Part print with two shaded views. Sizes in mm from the minimum x, y, z corner. A direction names the side the tool comes from. Give positions to 0.01 mm unless a question says otherwise; leave off trailing zeros. Order: outer loops, then holes, each group sorted by start corner. A loop starts at its lowest first (then second) coordinate and runs counter-clockwise, first axis right, second up. Notation, with made-up numbers: M -36,11.5 L -10,11.5 A23 cw -10,48.5 Z; hole C 21.25,65 d1. An arc over 180 degrees is marked long. Answer as CSV lines item,"result".
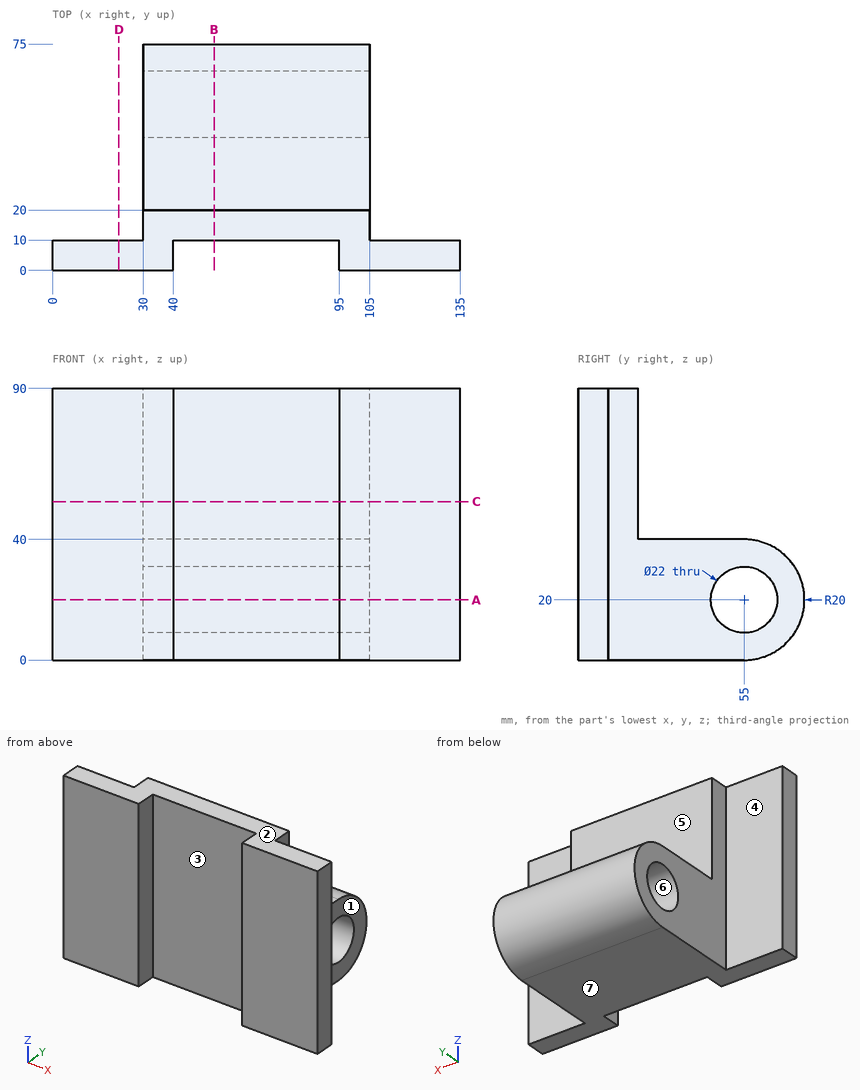
Item 1: Drop flat-ended pins along their axis: pin 1 (6 mm diameter, centred on x = 61.5, z = 57.5, fed in from +Y); pin 2 (8 mm diameter, centred on x = 102.5, y = 66, fed in from +Z) (3 decimals); pin 3 (8 mm diameter, centred on x = 86.5, y = 49, fed in from +Z). Give the stop position or say it passes through.
Geometry says:
pin 1,"stops at y = 20"
pin 2,"stops at z = 38.735"
pin 3,"stops at z = 40"
Item 2: Band-saw the part on A-A (z = 20). Give the cut face in (x, y), and give its area (4 significant figures).
Geometry says:
outline,"M 0,0 L 40,0 L 40,10 L 95,10 L 95,0 L 135,0 L 135,10 L 105,10 L 105,44 L 30,44 L 30,10 L 0,10 Z; M 30,66 L 105,66 L 105,75 L 30,75 Z"
area,"4,025 mm2"
Item 3: Pull direction Z, two halves, no side cores. Call the marked faces 5, 6 and 7: released by +Z, released by -Z, zero draft, split by the parting line, or undercut.
Geometry says:
face 5,"zero draft"
face 6,"undercut"
face 7,"released by -Z"
Item 4: Probe line 1 along Z through (x, y) = (85, 55); line 2 along Y through (x, z) = (54, 65); line 3 along X through (y, z) = (27.5, 28). List the from-to ranges inside material, lowest first. Write a range as from..to.
Geometry says:
line 1,"z = 0..9, 31..40"
line 2,"y = 10..20"
line 3,"x = 30..105"
Item 5: Band-saw the part on B-B (x = 53.5). Give the cut face in (y, z), and give its area (3 significant figures).
Geometry says:
outline,"M 10,0 L 55,0 A20 ccw 55,40 L 20,40 L 20,90 L 10,90 Z; hole C 55,20 d22"
area,"2,550 mm2"
Item 6: Band-saw the part on C-C (z = 52.5). Give the cut face in (x, y), and give its area (3 significant figures).
Geometry says:
outline,"M 0,0 L 40,0 L 40,10 L 95,10 L 95,0 L 135,0 L 135,10 L 105,10 L 105,20 L 30,20 L 30,10 L 0,10 Z"
area,"1,550 mm2"
Item 7: 3-axis set-ups, long thin cutter, end or side, ignore diameter. For the marked faces 1, 2, 3 and 4: which of +Z, -Z, +X, -X, +Y, -Y reach the whole face in a straight line?
Geometry says:
face 1,"+Z, -Z, +X, +Y"
face 2,"+Z, +X, -X, +Y, -Y"
face 3,"+Z, -Z, -Y"
face 4,"+Z, -Z, -X, +Y"
Item 8: Band-saw the part on D-D (x = 22). Give the cut face in (y, z).
Geometry says:
outline,"M 0,0 L 10,0 L 10,90 L 0,90 Z"
